CAD build for the part. Positions are in the model's coordinates, mm. A direction names the side the tool comes from. Coordinates: 2 decimals unless noted, no trailing zeros. Order: outer loops, then holes, each group sorted by start corner. A loop starts at its lowest first (then second) coordinate and runs counter-clockwise, first axis right, second up. Notation, with made-up numbers: (-0.5, 37) - (37.5, 37) arc R13 ccw to (37.5, 47) - close; hole circle Ø8 at (-37.5, 57). An arc over 180 degrees is marked (long way). Return JSON: item names as keys, results as strings.
from build123d import *

# Parameters (mm, degrees)
SKETCH2_R           = 2.85
BOSS_EXTRUDE1_DEPTH = 8
CHAMFER1_SIZE       = 0.5
BOSS_EXTRUDE3_START = -2
SKETCH4_R           = 1.6
BOSS_EXTRUDE3_DEPTH = 2


with BuildPart() as part:
    # Sketch2 → Boss-Extrude1 (new body)
    with BuildSketch(Plane(origin=(0, 0, 0), x_dir=(1, 0, 0), z_dir=(0, 1, 0))):
        with BuildLine():
            ThreePointArc((5, 0), (0, 5), (-5, 0))
            ThreePointArc((-5, 0), (-5.709068994, -3.199165875), (-7.703467842, -5.799130177))
            ThreePointArc((-7.703467842, -5.799130177), (-8.760764425, -17.760055771), (3.19780255, -18.843703794))
            ThreePointArc((3.19780255, -18.843703794), (4.527085859, -17.122614809), (5, -15))
            Line((5, -15), (5, 0))
        make_face()
        with Locations(Location((0, 0, 0), (0, 0, 270))):
            Circle(SKETCH2_R, mode=Mode.SUBTRACT)
    extrude(amount=BOSS_EXTRUDE1_DEPTH)

    # Chamfer1
    chamfer1_edges = [part.edges().sort_by_distance(p)[0] for p in [
        (0, 8, -2.85),
    ]]
    chamfer(chamfer1_edges, length=CHAMFER1_SIZE)

    # Sketch4 → Boss-Extrude3 (add)
    with BuildSketch(Plane(origin=(0, 0, 0), x_dir=(1, 0, 0), z_dir=(0, 1, 0)).offset(BOSS_EXTRUDE3_START)):
        with BuildLine():
            Line((5, -15), (5, 0))
            ThreePointArc((5, 0), (0, 5), (-5, 0))
            ThreePointArc((-5, 0), (-5.709068994, -3.199165875), (-7.703467842, -5.799130177))
            ThreePointArc((-7.703467842, -5.799130177), (-8.760764425, -17.760055771), (3.19780255, -18.843703794))
            ThreePointArc((3.19780255, -18.843703794), (4.527085859, -17.122614809), (5, -15))
        make_face()
        with Locations(Location((0, 0, 0), (0, 0, 270))):
            Circle(SKETCH4_R, mode=Mode.SUBTRACT)
    extrude(amount=BOSS_EXTRUDE3_DEPTH)


solid = part.part
Item 1: Band-saw the part on A-A, the plane x = 0. List the corners of the cut face in (y, z), then the cut area to 3 significant figures.
Findings below:
{"outline": "(-2, -5) - (8, -5) - (8, -3.35) - (7.5, -2.85) - (0, -2.85) - (0, -1.6) - (-2, -1.6) - close; (-2, 1.6) - (0, 1.6) - (0, 2.85) - (7.5, 2.85) - (8, 3.35) - (8, 20.51) - (-2, 20.51) - close", "area": "203 mm²"}
Item 2: Wall check: L1, parallel to X at y = 4, z = 0; L2, parallel to X at y = -0.8, z = 0; L3, parallel to Z at x = 0.25, y = 5. Give the ranges that are in metal, low to high. Write a range as [from, to].
Findings below:
{"L1": "x = [-5, -2.85], [2.85, 5]", "L2": "x = [-5, -1.6], [1.6, 5]", "L3": "z = [-4.99, -2.84], [2.84, 20.44]"}
Item 3: Drop a flat-ended pin along its axis: P1, Ø2, axis at x = -9, y = 2.5, coming from the -Z side. Give the stop position or say it passes through.
Findings below:
{"P1": "stops at z = 6.06"}
Item 4: Band-saw the part on D-D, the plane z = 15.5. List the corners of the cut face in (x, y), then the cut area to 3 significant figures.
Findings below:
{"outline": "(-10.12, -2) - (4.97, -2) - (4.97, 8) - (-10.12, 8) - close", "area": "151 mm²"}
Item 5: Band-saw the part on C-C, the plane x = -5.5. List the corners of the cut face in (y, z), then the cut area to 3 significant figures.
Findings below:
{"outline": "(-2, 2.71) - (8, 2.71) - (8, 20.16) - (-2, 20.16) - close", "area": "175 mm²"}
Item 6: Which spindle directions (+Z, -Z, +X, -X, +Y, -Y) get a long thin tool onto all of the face, cutting with end or side? Do faces 1 (the cylindrical face through (-1.734, 3.698, -2.262)), 2 (the cylindrical face through (-5.69, 2.93, 3.16)). Say none if no direction does.
Findings below:
{"face 1": "+Y", "face 2": "-Z, -X, +Y, -Y"}
Item 7: Mould opens along X. For faces 3 (the flat face through (0, 0, 2)), 4 (the cylindrical face through (-8.879, 2.93, 17.616)), 5 (the flat face through (-1, -2, 8)) say: released by +X, released by -X, zero draft, split by the parting line, or undercut.
Findings below:
{"face 3": "undercut", "face 4": "split by the parting line", "face 5": "zero draft"}
